The listing builds one solid part. Answer for the finished solid, in the listing's coordinates (mm). A direction names the side the tool comes from. Give positions to 0.01 mm unless a question says otherwise; leave off trailing zeros. Loops run counter-clockwise (first coordinate to the right, second up) from the corner with the lowest first, then second, coordinate; pieces in that order, holes last.
Item 1: Each of these flat-tipped pins is pushed along its axis until it touches: pin 1 Ø10 at (x, y) = (-6.5, 1) entering from +Z; pin 2 Ø12 at (y, z) = (0, 16) entering from +X. Where does it stop, or does it pass through?
Item 2: The mould has two halves that part along X. Classify faces 3 (the face through (0, 16, 73)), 4 (the face through (0, 14.4, 73)), 5 (the face through (-16, 0, 73)): pulls with the +X half, pulls with the -X half, needs draft (parallel to the pull), parting line crosses it, or undercut.
Item 3: Section B-B, the plane y = -10.5 is taken. Give the vertices of the cut face in (x, z).
Item 4: Section C-C, the plane z = 76.5 is taken. Give the vertices of the cut face in (x, y), and give its area (3 significant figures).
Item 5: A tool of negligible diameter and unlimited length cuts with its end or side. For faces 1 (the face through (0, -14.4, 73)), 2 (the face through (-15.211, -0.231, 21.245)), from which of +Z, -Z, +X, -X, +Y, -Y can it reach the whole face along a straight path? Write none if from no direction.
Item 6: Section A-A, the plane y = 0 is taken. Give the vertices of the cut face in (x, z), and give its area (3 significant figures).
Item 7: Consider line 1 along Y through (x, z) = (14.9, 16); line 2 along Y through (x, z) = (11, 136.5). Determine where each line is inside the solid, lowest interval first.
Autodesk Inventor part; units mm, degrees
ref_plane "YZ Plane" through (0, 0, 0) normal (1, 0, 0) x (0, 1, 0)
ref_plane "XZ Plane" through (0, 0, 0) normal (0, 1, 0) x (-1, 0, 0)
ref_plane "XY Plane" through (0, 0, 0) normal (0, 0, 1) x (1, 0, 0)
sketch "スケッチ1" plane through (0, 0, 0) normal (0, 0, 1) x (1, 0, 0)
  line L0 (-16, -16) -> (16, -16)
  line L1 (16, -16) -> (16, 16)
  line L2 (16, 16) -> (-16, 16)
  line L3 (-16, 16) -> (-16, -16)
  line L4 (-16, -16) -> (16, 16) construction
  line L5 (16, -16) -> (-16, 16) construction
  line L6 (-14.4, 14.4) -> (14.4, 14.4)
  line L7 (14.4, 14.4) -> (14.4, -14.4)
  line L8 (14.4, -14.4) -> (-14.4, -14.4)
  line L9 (-14.4, -14.4) -> (-14.4, 14.4)
  point P0 (0, 0)
  dimension "d0" = 32
  dimension "d1" = 32
  dimension "d2" = 1.6
extrude "押し出し1" add sketch "スケッチ1" along normal blind 147.5
sketch "スケッチ2" plane through (16, -16, 147.5) normal (1, 0, 0) x (0, 0, -1)
  line L0 (0, 0) -> (0, 32)
  point P0 (147.5, 16)
  point P1 (131.5, 16)
  dimension "d8" = 131.5
hole "穴1" at (16, 0, 16) direction (-1, 0, 0) diameter 10.5 end through all
properties part number "PipeB"
Worked answers:
1. pin 1: passes through
1. pin 2: stops at x = 16
2. face 3: needs draft
2. face 4: undercut
2. face 5: pulls with the -X half
3. outline: (-16, 0) - (-14.4, 0) - (-14.4, 147.5) - (-16, 147.5) - close; (14.4, 0) - (16, 0) - (16, 147.5) - (14.4, 147.5) - close
4. outline: (-16, -16) - (16, -16) - (16, 16) - (-16, 16) - close; hole (-14.4, -14.4) - (14.4, -14.4) - (14.4, 14.4) - (-14.4, 14.4) - close
4. area: 195 mm2
5. face 1: +Z, -Z
5. face 2: +X, -X
6. outline: (-16, 0) - (-14.4, 0) - (-14.4, 10.75) - (-16, 10.75) - close; (-16, 21.25) - (-14.4, 21.25) - (-14.4, 147.5) - (-16, 147.5) - close; (14.4, 0) - (16, 0) - (16, 10.75) - (14.4, 10.75) - close; (14.4, 21.25) - (16, 21.25) - (16, 147.5) - (14.4, 147.5) - close
6. area: 438 mm2
7. line 1: y = -16 to -5.25, 5.25 to 16
7. line 2: y = -16 to -14.4, 14.4 to 16
